Check sheet for the modelled part. Datum: model origin and axes. Units: mm. Face numbers are marked on the shaded views. Coordinates: 2 decimals unless noted, no trailing zeros. Loops run counter-clockwise (first coordinate to the right, second up) from the corner with the lowest first, then second, coordinate; pieces in that order, holes last.
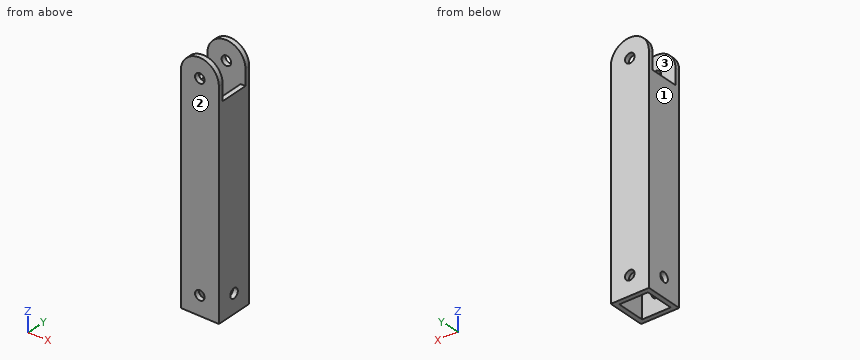
Autodesk Inventor part; units mm, degrees
ref_plane "YZ Plane" through (0, 0, 0) normal (1, 0, 0) x (0, 1, 0)
ref_plane "XZ Plane" through (0, 0, 0) normal (0, 1, 0) x (-1, 0, 0)
ref_plane "XY Plane" through (0, 0, 0) normal (0, 0, 1) x (1, 0, 0)
sketch "Sketch1" plane through (0, 0, 0) normal (0, 0, 1) x (1, 0, 0)
  line L0 (0, 0) -> (25.4, 0)
  line L1 (25.4, 0) -> (25.4, 25.4)
  line L2 (25.4, 25.4) -> (0, 25.4)
  line L3 (0, 25.4) -> (0, 0)
  line L4 (3.175, 3.175) -> (22.225, 3.175)
  line L5 (22.225, 3.175) -> (22.225, 22.225)
  line L6 (22.225, 22.225) -> (3.175, 22.225)
  line L7 (3.175, 22.225) -> (3.175, 3.175)
  dimension "d0" = 3.175
  dimension "d1" = 3.175
  dimension "d2" = 3.175
  dimension "d3" = 3.175
  dimension "d4" = 25.4
  dimension "d5" = 25.4
extrude "Extrusion1" add sketch "Sketch1" along normal blind 158.75
sketch "Sketch2" plane through (0, 25.4, 0) normal (0, 1, 0) x (1, 0, 0)
  line L0 (0, -158.75) -> (25.4, -158.75)
  line L1 (25.4, 0) -> (25.4, -158.75)
  line L2 (25.4, 0) -> (0, 0)
  line L3 (0, 0) -> (0, -158.75)
  circle A0 centre (12.7, -146.05) radius 3.175
  arc A1 (0, -146.05) -> (25.4, -146.05) centre (12.7, -146.05) ccw
  circle A2 centre (12.7, -12.7) radius 3.175
  point P0 (12.7, 0)
  dimension "d8" = 6.35
  dimension "d17" = 12.7
  dimension "d18" = 6.35
extrude "Extrusion2" cut sketch "Sketch2" against normal through all contours L3 A1 L0 | A1 L1 L0 | A0 | A2
sketch "Sketch3" plane through (25.4, 0, 0) normal (1, 0, 0) x (0, 0, -1)
  line L0 (0, 0) -> (0, 25.4)
  line L1 (0, 25.4) -> (-146.05, 25.4)
  line L2 (-154.4503, 3.175) -> (-154.4503, 22.225)
  line L3 (-154.4503, 22.225) -> (-135.4003, 22.225)
  line L4 (-135.4003, 22.225) -> (-135.4003, 3.175)
  line L5 (-135.4003, 3.175) -> (-154.4503, 3.175)
  line L6 (-154.4503, 3.175) -> (-154.4503, 22.225)
  circle A0 centre (-12.7, 12.7) radius 3.175
  dimension "d11" = 19.05
  dimension "d12" = 6.35
  dimension "d13" = 12.7
  dimension "d14" = 12.7
extrude "Extrusion3" cut sketch "Sketch3" against normal through all
equation "\"d0\" = d3"
equation "\"d1\" = d3"
equation "\"d2\" = d1"
equation "\"d18\" = d8"
properties part number "pnumatic arm lever"
1) Section check A-A on z = 138.5. Enter the section's corners in (x, y) (3 decimals).
Answer sheet:
outline: (0, 0) - (25.4, 0) - (25.4, 3.175) - (0, 3.175) - close; (0, 22.225) - (25.4, 22.225) - (25.4, 25.4) - (0, 25.4) - close
2) Depth check by flat-ended pin: pin 1 (8 mm diameter, centred on x = 5, y = 2.5, fed in from +Z); pin 2 (1 mm diameter, centred on x = 2, y = 11, fed in from +Z). Enter the tip coordinate at first touch or a pass-through.
Answer sheet:
pin 1: stops at z = 158.2
pin 2: stops at z = 135.4
3) Section check B-B on x = 12.7. Enter the section's corners in (y, z) (3 decimals).
Answer sheet:
outline: (0, 0) - (3.175, 0) - (3.175, 9.525) - (0, 9.525) - close; (0, 15.875) - (3.175, 15.875) - (3.175, 142.875) - (0, 142.875) - close; (0, 149.225) - (3.175, 149.225) - (3.175, 158.75) - (0, 158.75) - close; (22.225, 0) - (25.4, 0) - (25.4, 9.525) - (22.225, 9.525) - close; (22.225, 15.875) - (25.4, 15.875) - (25.4, 142.875) - (22.225, 142.875) - close; (22.225, 149.225) - (25.4, 149.225) - (25.4, 158.75) - (22.225, 158.75) - close
4) Scan lines: line 1 (Z direction, x = 12.7, y = 23.65) (3 decimals); line 2 (Y direction, x = 24.45, z = 12.7) (3 decimals). Record each from-to range of solid material in increasing order.
Answer sheet:
line 1: z = 0 to 9.525, 15.875 to 142.875, 149.225 to 158.75
line 2: y = 0 to 9.525, 15.875 to 25.4
5) Mould release check, pull along X, two halves, no side actions. Record for the marked faces 1, 2 and 3: +X half, -X half, draft (parallel to the pull), parting line (faces both ways), or undercut.
Answer sheet:
face 1: -X half
face 2: draft
face 3: undercut
6) Section check C-C on z = 12.7. Enter the section's corners in (x, y) (3 decimals).
Answer sheet:
outline: (0, 0) - (9.525, 0) - (9.525, 3.175) - (3.175, 3.175) - (3.175, 9.525) - (0, 9.525) - close; (0, 15.875) - (3.175, 15.875) - (3.175, 22.225) - (9.525, 22.225) - (9.525, 25.4) - (0, 25.4) - close; (15.875, 0) - (25.4, 0) - (25.4, 9.525) - (22.225, 9.525) - (22.225, 3.175) - (15.875, 3.175) - close; (15.875, 22.225) - (22.225, 22.225) - (22.225, 15.875) - (25.4, 15.875) - (25.4, 25.4) - (15.875, 25.4) - close
7) Section check D-D on y = 12.7. Enter the section's corners in (x, z) (3 decimals).
Answer sheet:
outline: (0, 0) - (3.175, 0) - (3.175, 9.525) - (0, 9.525) - close; (0, 15.875) - (3.175, 15.875) - (3.175, 135.4) - (0, 135.4) - close; (22.225, 0) - (25.4, 0) - (25.4, 9.525) - (22.225, 9.525) - close; (22.225, 15.875) - (25.4, 15.875) - (25.4, 135.4) - (22.225, 135.4) - close
